Source: CAD feature listing. Evaluate the final solid. Frame: model axes, mm. A direction names the side the tool comes from. Coordinates: 2 decimals unless noted, no trailing zeros. Order: outer loops, then holes, each group sorted by start corner. A loop starts at its lowest first (then second) coordinate and runs counter-clockwise, first axis right, second up.
```python
from build123d import *

# Parameters (mm, degrees)
SKETCH1_R           = 3.175
SKETCH1_R_2         = 6.35
SKETCH1_R_3         = 1.5875
BOSS_EXTRUDE1_DEPTH = 25.4
CUT_EXTRUDE1_REACH  = 40.1
SKETCH2_W           = 12.7
SKETCH2_H           = 44.958
CUT_EXTRUDE2_REACH  = 27.4
SKETCH3_R           = 1.651
BOSS_EXTRUDE2_DEPTH = 38.1
BOSS_EXTRUDE3_DEPTH = 12.7
BOSS_EXTRUDE4_DEPTH = 3.175


with BuildPart() as part:
    # Sketch1 → Boss-Extrude1 (new body)
    with BuildSketch(Plane.XY):
        with BuildLine():
            Line((-19.05, 50.8), (-19.05, -50.8))
            ThreePointArc((-19.05, -50.8), (0, -69.85), (19.05, -50.8))
            Line((19.05, -50.8), (19.05, 50.8))
            ThreePointArc((19.05, 50.8), (0, 69.85), (-19.05, 50.8))
        make_face()
        with Locations((0, 50.8)):
            Circle(SKETCH1_R, mode=Mode.SUBTRACT)
        with Locations((0, -50.8)):
            Circle(SKETCH1_R_2, mode=Mode.SUBTRACT)
        with Locations((0, 63.5)):
            Circle(SKETCH1_R_3, mode=Mode.SUBTRACT)
        with Locations((-12.7, 50.8)):
            Circle(SKETCH1_R_3, mode=Mode.SUBTRACT)
        with Locations((0, 38.1)):
            Circle(SKETCH1_R_3, mode=Mode.SUBTRACT)
        with Locations((12.7, 50.8)):
            Circle(SKETCH1_R_3, mode=Mode.SUBTRACT)
    extrude(amount=BOSS_EXTRUDE1_DEPTH)

    # Sketch2 → Cut-Extrude1 (cut, up to next)
    with BuildSketch(Plane(origin=(19.05, 0, 0), x_dir=(0, 0, -1), z_dir=(1, 0, 0)), mode=Mode.PRIVATE) as cut_extrude1_sk1:
        with Locations((-6.35, 47.371)):
            Rectangle(SKETCH2_W, SKETCH2_H)
    cut_extrude1_tool1 = extrude(cut_extrude1_sk1.sketch, amount=-CUT_EXTRUDE1_REACH, mode=Mode.PRIVATE) & part.part
    add(cut_extrude1_tool1.solids().sort_by_distance((19.05, 47.371, 6.35))[0], mode=Mode.SUBTRACT)
    # Sketch2 → Cut-Extrude1 (cut, up to next)
    with BuildSketch(Plane(origin=(19.05, 0, 0), x_dir=(0, 0, -1), z_dir=(1, 0, 0)), mode=Mode.PRIVATE) as cut_extrude1_sk2:
        with Locations((-6.35, -47.371)):
            Rectangle(SKETCH2_W, SKETCH2_H)
    cut_extrude1_tool2 = extrude(cut_extrude1_sk2.sketch, amount=-CUT_EXTRUDE1_REACH, mode=Mode.PRIVATE) & part.part
    add(cut_extrude1_tool2.solids().sort_by_distance((19.05, -47.371, 6.35))[0], mode=Mode.SUBTRACT)

    # Sketch3 → Cut-Extrude2 (cut, up to next)
    with BuildSketch(Plane(origin=(0, 0, 0), x_dir=(-1, 0, 0), z_dir=(0, 0, -1)), mode=Mode.PRIVATE) as cut_extrude2_sk1:
        with Locations((-7.62, -30.197275928)):
            Circle(SKETCH3_R)
    cut_extrude2_tool1 = extrude(cut_extrude2_sk1.sketch, amount=-CUT_EXTRUDE2_REACH, mode=Mode.PRIVATE) & part.part
    add(cut_extrude2_tool1.solids().sort_by_distance((7.62, -30.197276, 0))[0], mode=Mode.SUBTRACT)
    # Sketch3 → Cut-Extrude2 (cut, up to next)
    with BuildSketch(Plane(origin=(0, 0, 0), x_dir=(-1, 0, 0), z_dir=(0, 0, -1)), mode=Mode.PRIVATE) as cut_extrude2_sk2:
        with Locations((-15.24, -43.688)):
            Circle(SKETCH3_R)
    cut_extrude2_tool2 = extrude(cut_extrude2_sk2.sketch, amount=-CUT_EXTRUDE2_REACH, mode=Mode.PRIVATE) & part.part
    add(cut_extrude2_tool2.solids().sort_by_distance((15.24, -43.688, 0))[0], mode=Mode.SUBTRACT)
    # Sketch3 → Cut-Extrude2 (cut, up to next)
    with BuildSketch(Plane(origin=(0, 0, 0), x_dir=(-1, 0, 0), z_dir=(0, 0, -1)), mode=Mode.PRIVATE) as cut_extrude2_sk3:
        with Locations((-7.62, -57.178724072)):
            Circle(SKETCH3_R)
    cut_extrude2_tool3 = extrude(cut_extrude2_sk3.sketch, amount=-CUT_EXTRUDE2_REACH, mode=Mode.PRIVATE) & part.part
    add(cut_extrude2_tool3.solids().sort_by_distance((7.62, -57.178724, 0))[0], mode=Mode.SUBTRACT)
    # Sketch3 → Cut-Extrude2 (cut, up to next)
    with BuildSketch(Plane(origin=(0, 0, 0), x_dir=(-1, 0, 0), z_dir=(0, 0, -1)), mode=Mode.PRIVATE) as cut_extrude2_sk4:
        with Locations((7.62, -57.178724072)):
            Circle(SKETCH3_R)
    cut_extrude2_tool4 = extrude(cut_extrude2_sk4.sketch, amount=-CUT_EXTRUDE2_REACH, mode=Mode.PRIVATE) & part.part
    add(cut_extrude2_tool4.solids().sort_by_distance((-7.62, -57.178724, 0))[0], mode=Mode.SUBTRACT)
    # Sketch3 → Cut-Extrude2 (cut, up to next)
    with BuildSketch(Plane(origin=(0, 0, 0), x_dir=(-1, 0, 0), z_dir=(0, 0, -1)), mode=Mode.PRIVATE) as cut_extrude2_sk5:
        with Locations((15.24, -43.688)):
            Circle(SKETCH3_R)
    cut_extrude2_tool5 = extrude(cut_extrude2_sk5.sketch, amount=-CUT_EXTRUDE2_REACH, mode=Mode.PRIVATE) & part.part
    add(cut_extrude2_tool5.solids().sort_by_distance((-15.24, -43.688, 0))[0], mode=Mode.SUBTRACT)
    # Sketch3 → Cut-Extrude2 (cut, up to next)
    with BuildSketch(Plane(origin=(0, 0, 0), x_dir=(-1, 0, 0), z_dir=(0, 0, -1)), mode=Mode.PRIVATE) as cut_extrude2_sk6:
        with Locations((7.62, -30.197275928)):
            Circle(SKETCH3_R)
    cut_extrude2_tool6 = extrude(cut_extrude2_sk6.sketch, amount=-CUT_EXTRUDE2_REACH, mode=Mode.PRIVATE) & part.part
    add(cut_extrude2_tool6.solids().sort_by_distance((-7.62, -30.197276, 0))[0], mode=Mode.SUBTRACT)

    # Sketch5 → Boss-Extrude2 (add)
    with BuildSketch(Plane(origin=(0, 0, 0), x_dir=(-1, 0, 0), z_dir=(0, 0, -1))):
        with BuildLine():
            Line((-19.05, -41.097979346), (-19.05, -24.892))
            ThreePointArc((-19.05, -24.892), (0, -16.926234064), (19.05, -24.892))
            Line((19.05, -24.892), (19.05, -41.148))
            Line((19.05, -41.148), (18.324802864, -41.148))
            ThreePointArc((18.324802864, -41.148), (0, -25.188), (-18.324802864, -41.148))
            ThreePointArc((-18.324802864, -41.148), (-18.686539909, -41.110499348), (-19.05, -41.097979346))
        make_face()
    extrude(amount=BOSS_EXTRUDE2_DEPTH)

    # Sketch6 → Boss-Extrude3 (add)
    with BuildSketch(Plane.XY):
        with BuildLine():
            Line((-19.05, -24.892), (-19.05, -41.148))
            Line((-19.05, -41.148), (-18.324802864, -41.148))
            ThreePointArc((-18.324802864, -41.148), (0, -25.188), (18.324802864, -41.148))
            Line((18.324802864, -41.148), (19.05, -41.097979346))
            Line((19.05, -41.097979346), (19.05, -24.892))
            Line((19.05, -24.892), (-19.05, -24.892))
        make_face()
    extrude(amount=BOSS_EXTRUDE3_DEPTH)

    # Sketch7 → Boss-Extrude4 (add, symmetric)
    with BuildSketch(Plane(origin=(0, 0, 0), x_dir=(0, 0, -1), z_dir=(1, 0, 0))):
        Polygon((0, -19.466234064), (0, 5.933765936), (25.4, -19.466234064), align=None)
    extrude(amount=BOSS_EXTRUDE4_DEPTH, both=True)


solid = part.part
```
1. Section query A-A, the plane x = 0. Count the separate pieces of the cut face and the enclosed holes in it, plus the area to 3 significant figures.
2. Draft query along Y for faces 1 (the cylindrical face through (-0.419, -69.845, 18.961)), 2 (the flat face through (3.175, -11, -7)), 3 (the cylindrical face through (-7.41, -28.56, 18.96)). Return one class per face: +Y half, -Y half, draft (parallel to the pull), parting line (faces both ways), or undercut.
3. Material intervals for line 1 along X through (y, z) = (38.1, 18); line 2 along X through (y, z) = (-50.8, 17.5); line 3 along Z through (x, y) = (-7.5, 6), sorted ascending.
4. Section query C-C, the plane z = -21.5. Output: boundary loops of the cut face in (x, y) (3 decimals).
5. Section query B-B, the plane y = 38.1. Output: boundary loops of the cut face in (x, z).
6. Section query D-D, the plane x = 7.62. Output: boundary loops of the cut face in (y, z), plus the area to 3 significant figures.
7. Access query for faces 4 (the flat face through (-3.175, -11, -7)), 5 (the cylindrical face through (-0.37, -25.19, -13.06)), 6 (the flat face through (-5, 0, 0)). Directions: +Z, -Z, +X, -X, +Y, -Y. A direction counts if a zero-diameter tool reaches every point of the face in a straight line with its end or side. Return the directions, or none.
8. Contact query for flat-ended pins moving along their axis: P1, Ø2, axis at x = 1.5, z = -29, coming from the +Y side; P2, Ø6.5, axis at x = -6.5, z = 6, coming from the +Y side; P3, Ø19, axis at x = -4, y = 57.5, coming from the -Z side. Output: stop coordinate, or through.
Answer key:
1. separate pieces: 5
1. enclosed holes: 0
1. area: 2,660 mm2
2. face 1: -Y half
2. face 2: draft
2. face 3: undercut
3. line 1: x = -19.05 to -1.59, 1.59 to 19.05
3. line 2: x = -19.05 to -6.35, 6.35 to 19.05
3. line 3: z = 0 to 25.4
4. outline: (-19.05, -41.148) - (-18.325, -41.148) arc R18.5 cw to (18.325, -41.148) arc R5.282 cw to (19.05, -41.098) - (19.05, -24.892) arc R26.762 ccw to (3.175, -17.115) - (3.175, -15.566) - (-3.175, -15.566) - (-3.175, -17.115) arc R26.762 ccw to (-19.05, -24.892) - close
5. outline: (-19.05, 12.7) - (-1.59, 12.7) - (-1.59, 25.4) - (-19.05, 25.4) - close; (1.59, 12.7) - (19.05, 12.7) - (19.05, 25.4) - (1.59, 25.4) - close
6. outline: (-68.26, 12.7) - (-58.83, 12.7) - (-58.83, 25.4) - (-68.26, 25.4) - close; (-55.53, 12.7) - (-31.85, 12.7) - (-31.85, 25.4) - (-55.53, 25.4) - close; (-28.55, 12.7) - (-26.83, 12.7) - (-26.83, -38.1) - (-18.03, -38.1) - (-18.03, 0) - (24.89, 0) - (24.89, 12.7) - (68.26, 12.7) - (68.26, 25.4) - (-28.55, 25.4) - close
6. area: 2,640 mm2
7. face 4: -Z, -X, +Y
7. face 5: -Z, -Y
7. face 6: -Z, +Y
8. P1: stops at y = -16.93
8. P2: stops at y = 24.89
8. P3: stops at z = 12.7
